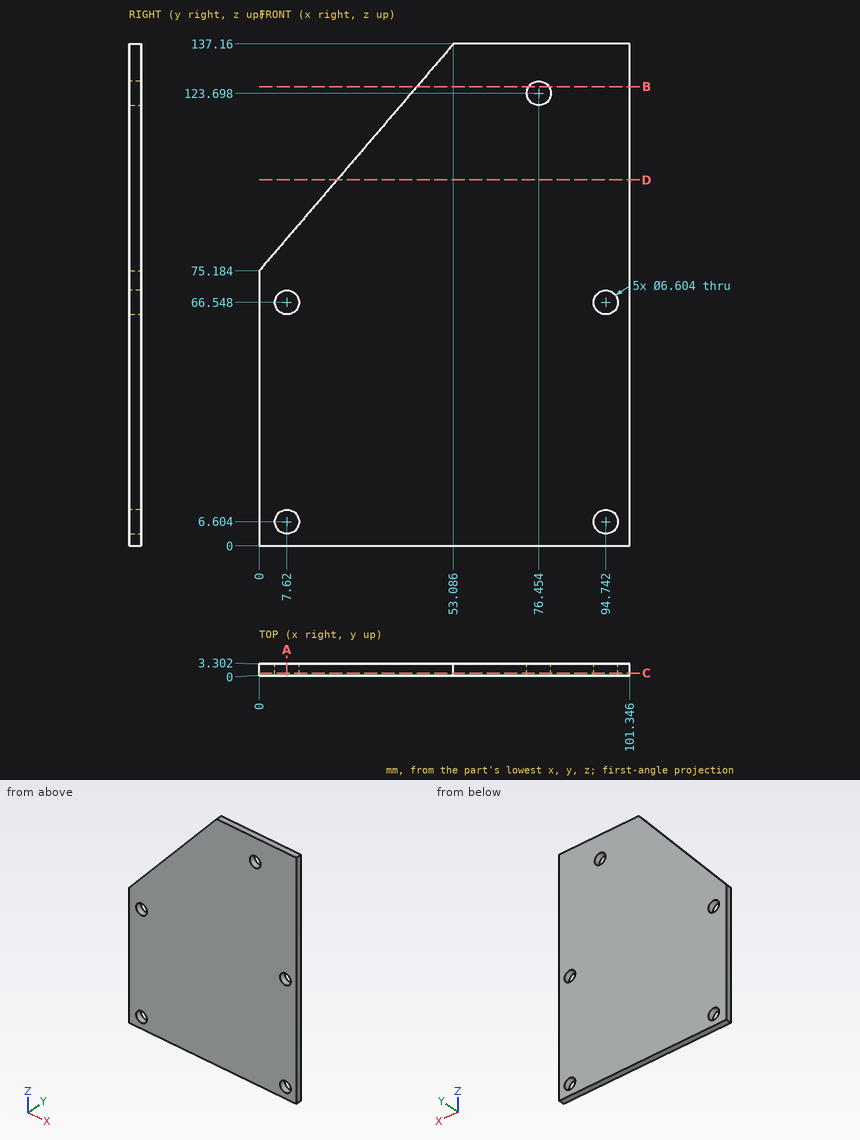
Verification items for this drawing (mm, ordinates from the low corner). Coordinates: 2 decimals unless noted, no trailing zeros. Write each loop counter-clockwise with the first axis right and the second up, starting at its lowest first coordinate (ties: lowest second). Pieces come first, ordered by that corner, then holes. Notation, with made-up numbers: M 37.25,-7 L 49.25,-7 A36 ccw 49.25,28 Z; hole C -14.75,29.25 d4. An arc over 180 degrees is marked long. Use CSV: the item, a comma, the result in double quotes.
Q1. Section check C-C, the plane y = 0.8. Enter the section's corners in (x, z), and give its area (3 significant figures).
Computed values:
outline,"M 0,0 L 101.35,0 L 101.35,137.16 L 53.09,137.16 L 0,75.18 Z; hole C 7.62,6.6 d6.6; hole C 7.62,66.55 d6.6; hole C 76.45,123.7 d6.6; hole C 94.74,6.6 d6.6; hole C 94.74,66.55 d6.6"
area,"12,100 mm²"
Q2. Thickness scan on line 1 along X through (y, z) = (1.75, 65.5); line 2 along X through (y, z) = (2.45, 121); line 3 along Z through (x, y) = (29, 0.3). Record the ranges inside material, lowest first. Write a range as [from, to].
Computed values:
line 1,"[0, 4.49], [10.75, 91.61], [97.87, 101.35]"
line 2,"[39.24, 74.55], [78.36, 101.35]"
line 3,"[0, 109.04]"
Q3. Section check B-B, the plane z = 125.5. Enter the section's corners in (x, y).
Computed values:
outline,"M 43.1,0 L 73.69,0 L 73.69,3.3 L 43.1,3.3 Z; M 79.22,0 L 101.35,0 L 101.35,3.3 L 79.22,3.3 Z"
Q4. Go/stop test with a flat-tipped pin: P1, Ø5.5, axis at x = 7.62, z = 66.548, coming from the -Y side. Record where the tip stops, or that it passes through.
Computed values:
P1,"through"
Q5. Section check D-D, the plane z = 100. Enter the section's corners in (x, y).
Computed values:
outline,"M 21.26,0 L 101.35,0 L 101.35,3.3 L 21.26,3.3 Z"
Q6. Section check A-A, the plane x = 7.62. Enter the section's corners in (y, z), and give its area (3 significant figures).
Computed values:
outline,"M 0,0 L 3.3,0 L 3.3,3.3 L 0,3.3 Z; M 0,9.91 L 3.3,9.91 L 3.3,63.25 L 0,63.25 Z; M 0,69.85 L 3.3,69.85 L 3.3,84.08 L 0,84.08 Z"
area,"234 mm²"
